Read the model definition and answer for the solid it produces. Units are mm, in the model's axes. A direction names the side the tool comes from. Coordinates: 2 decimals unless noted, no trailing zeros. Loops run counter-clockwise (first coordinate to the right, second up) from the corner with the lowest first, then second, coordinate; pieces in that order, holes last.
from build123d import *

# Parameters (mm, degrees)
SKETCH1_W           = 50.8
SKETCH1_H           = 25.4
SKETCH1_W_2         = 47.625
SKETCH1_H_2         = 22.225
BOSS_EXTRUDE1_DEPTH = 63.5
SKETCH2_R           = 2.4892
CUT_EXTRUDE1_DEPTH  = 26.4
SKETCH3_R           = 2.4892
CUT_EXTRUDE2_DEPTH  = 51.8


with BuildPart() as part:
    # Sketch1 → Boss-Extrude1 (new body, symmetric)
    with BuildSketch(Plane.XY):
        Rectangle(SKETCH1_W, SKETCH1_H)
        Rectangle(SKETCH1_W_2, SKETCH1_H_2, mode=Mode.SUBTRACT)
    extrude(amount=BOSS_EXTRUDE1_DEPTH, both=True)

    # Sketch2 → Cut-Extrude1 (cut, through all)
    with BuildSketch(Plane(origin=(0, 12.7, 0), x_dir=(1, 0, 0), z_dir=(0, 1, 0))):
        with Locations((-12.7, 50.8)):
            Circle(SKETCH2_R)
        with Locations((0, 50.8)):
            Circle(SKETCH2_R)
        with Locations((12.7, 50.8)):
            Circle(SKETCH2_R)
        with Locations((12.7, -50.8)):
            Circle(SKETCH2_R)
        with Locations((0, -50.8)):
            Circle(SKETCH2_R)
        with Locations((-12.7, -50.8)):
            Circle(SKETCH2_R)
    extrude(amount=-CUT_EXTRUDE1_DEPTH, mode=Mode.SUBTRACT)

    # Sketch3 → Cut-Extrude2 (cut, through all)
    with BuildSketch(Plane(origin=(25.4, 0, 0), x_dir=(0, 0, -1), z_dir=(1, 0, 0))):
        with Locations((50.8, 0)):
            Circle(SKETCH3_R)
        with Locations((41.275, 0)):
            Circle(SKETCH3_R)
        with Locations((15.875, 0)):
            Circle(SKETCH3_R)
        with Locations((-50.8, 0)):
            Circle(SKETCH3_R)
        with Locations((-31.75, 0)):
            Circle(SKETCH3_R)
        with Locations((-15.875, 0)):
            Circle(SKETCH3_R)
    extrude(amount=-CUT_EXTRUDE2_DEPTH, mode=Mode.SUBTRACT)


solid = part.part
Item 1: A cutting plane is placed at C-C on x = 12.7. Determine the outline of the cut face in (y, z).
Numbers:
outline: (-12.7, -63.5) - (-11.11, -63.5) - (-11.11, -53.29) - (-12.7, -53.29) - close; (-12.7, -48.31) - (-11.11, -48.31) - (-11.11, 48.31) - (-12.7, 48.31) - close; (-12.7, 53.29) - (-11.11, 53.29) - (-11.11, 63.5) - (-12.7, 63.5) - close; (11.11, -63.5) - (12.7, -63.5) - (12.7, -53.29) - (11.11, -53.29) - close; (11.11, -48.31) - (12.7, -48.31) - (12.7, 48.31) - (11.11, 48.31) - close; (11.11, 53.29) - (12.7, 53.29) - (12.7, 63.5) - (11.11, 63.5) - close
Item 2: A cutting plane is placed at D-D on x = -18.5. Determine the outline of the cut face in (y, z), then the cut area to 3 significant figures.
Numbers:
outline: (-12.7, -63.5) - (-11.11, -63.5) - (-11.11, 63.5) - (-12.7, 63.5) - close; (11.11, -63.5) - (12.7, -63.5) - (12.7, 63.5) - (11.11, 63.5) - close
area: 403 mm2
Item 3: A cutting plane is placed at A-A on z = -33. Determine the outline of the cut face in (x, y).
Numbers:
outline: (-25.4, -12.7) - (25.4, -12.7) - (25.4, 12.7) - (-25.4, 12.7) - close; hole (-23.81, -11.11) - (23.81, -11.11) - (23.81, 11.11) - (-23.81, 11.11) - close
Item 4: Find the intervals of material crossed by line 1 along Z through (x, y) = (-12.7, 12.35); line 2 along Y through (x, z) = (-3, 6.5); line 3 along X through (y, z) = (2.5, 11.5), in increasing order.
Numbers:
line 1: z = -63.5 to -53.29, -48.31 to 48.31, 53.29 to 63.5
line 2: y = -12.7 to -11.11, 11.11 to 12.7
line 3: x = -25.4 to -23.81, 23.81 to 25.4
Item 5: Determine the mould class of faces 3 (the face through (-0.54, -11.9, 53.23)), 4 (the face through (25.4, 0, 1)), 5 (the face through (0, -12, 63.5)), 6 (the face through (-25.4, 0, 1)) for opening direction X: released by +X, released by -X, zero draft, split by the parting line, or undercut.
Numbers:
face 3: undercut
face 4: released by +X
face 5: zero draft
face 6: released by -X
Item 6: A cutting plane is placed at B-B on y = 7.75. Determine the outline of the cut face in (x, z).
Numbers:
outline: (-25.4, -63.5) - (-23.81, -63.5) - (-23.81, 63.5) - (-25.4, 63.5) - close; (23.81, -63.5) - (25.4, -63.5) - (25.4, 63.5) - (23.81, 63.5) - close
Item 7: Which of the six approach directions +Z, -Z, +X, -X, +Y, -Y give full straight-line access (tool end or side, diameter ignored) to faces 1 (the face through (-24.595, 0.109, 34.237)), 2 (the face through (0, 11.112, 1))?
Numbers:
face 1: +X, -X
face 2: +Z, -Z
